Here's how the part is built. I have some questions about the finished solid (model axes, mm). A direction names the side the tool comes from. Give positions to 0.01 mm unless a question says otherwise; leave off trailing zeros. Write each loop counter-clockwise with the first axis right and the second up, starting at its lowest first coordinate (ties: lowest second). Pieces come first, ordered by that corner, then holes. Notation, with made-up numbers: (48.5, 70.25) - (53.5, 70.25) arc R24 ccw to (53.5, 105.25) - close; hole circle Ø9 at (-3, 46.25). An arc over 180 degrees is marked (long way). Use a Markdown table: item, result.
```python
from build123d import *

# Parameters (mm, degrees)
SKETCH1_W                  = 127.078191072
SKETCH1_H                  = 113.282646321
BOSS_EXTRUDE1_DEPTH        = 39.624
SHELL_1_T                  = -2.54
OFFICIAL_RIB_BLOCK20_REACH = 100.208


with BuildPart() as part:
    # Sketch1 → Boss-Extrude1 (new body)
    with BuildSketch(Plane(origin=(0, 0, 0), x_dir=(1, 0, 0), z_dir=(0, 1, 0))):
        with Locations((1.06119575, 7.295720781)):
            Rectangle(SKETCH1_W, SKETCH1_H)
    extrude(amount=BOSS_EXTRUDE1_DEPTH)

    # 抽壳1
    shell_1_openings = [part.faces().sort_by_distance(p)[0] for p in [
        (1.06119575, 39.624, -7.295720782),
    ]]
    offset(amount=SHELL_1_T, openings=shell_1_openings, kind=Kind.INTERSECTION)

    # 草图1 walls → official_rib_block20 (add, up to next)
    with BuildSketch(Plane(origin=(0.729572078, 0, -0.729572078), x_dir=(0.7071067811865477, 0, 0.7071067811865475), z_dir=(-0.7071067811865475, 0, 0.7071067811865477)), mode=Mode.PRIVATE) as official_rib_block20_sk1:
        Polygon((-181.514338156, -5.000960726), (-34.23, 35.134), (7.726, 25.357), (209.797270961, 53.134303954), (209.451367988, 55.650640802), (7.84521248, 27.93727297), (-34.278590113, 37.753375981), (-182.182137615, -2.550319201), align=None)
    official_rib_block20_tool1 = extrude(official_rib_block20_sk1.sketch, amount=-OFFICIAL_RIB_BLOCK20_REACH, mode=Mode.PRIVATE) - part.part
    add(official_rib_block20_tool1.solids().sort_by_distance((-8.641006986, 30.2455, -10.100151142))[0])


solid = part.part
```
Item 1: For faces 5 (the flat face through (64.6, 20, -7)), 6 (the flat face through (46.229, 28.993, 2.099)), 7 (the flat face through (-23.509, 32.392, -52.792)), which set-ups out of +Z, -Z, +X, -X, +Y, -Y let a thin tool reach every point of the face, with its end or its side?
Values:
| item | result |
|---|---|
| face 5 | +Z, -Z, +X, +Y, -Y |
| face 6 | none |
| face 7 | +Y |
Item 2: If we section it at D-D, the plane z = -17.5: Write out the boundary of the cut face in (x, y).
Values:
| item | result |
|---|---|
| outline | (-62.48, 0) - (64.6, 0) - (64.6, 39.62) - (62.06, 39.62) - (62.06, 31.19) - (28.59, 27.94) - (-16.04, 35.29) - (-16.04, 32.68) - (28.43, 25.36) - (62.06, 28.63) - (62.06, 2.54) - (-59.94, 2.54) - (-59.94, 39.62) - (-62.48, 39.62) - close |
Item 3: Will this pin go through, and if not, where does the flat tip stop? pin 1 Ø1 at (x, z) = (-26, -29) entering from +Y.
Values:
| item | result |
|---|---|
| pin 1 | stops at y = 36.63 |
Item 4: If we section it at A-A, the plane y = 7.5: Write out the boundary of the cut face in (x, z).
Values:
| item | result |
|---|---|
| outline | (-62.48, -63.94) - (64.6, -63.94) - (64.6, 49.35) - (-62.48, 49.35) - close; hole (-59.94, -61.4) - (62.06, -61.4) - (62.06, 46.81) - (-59.94, 46.81) - close |
Item 5: If we section it at B-B, the plane z = 9.5: Write out the boundary of the cut face in (x, y).
Values:
| item | result |
|---|---|
| outline | (-62.48, 0) - (64.6, 0) - (64.6, 39.62) - (62.06, 39.62) - (62.06, 33.81) - (10.96, 28.85) - (10.96, 26.28) - (62.06, 31.25) - (62.06, 2.54) - (-59.94, 2.54) - (-59.94, 39.62) - (-62.48, 39.62) - close |
Item 6: I need wall thicknesses on line 1 along X through (y, z) = (31, 42); line 2 along Z through (x, y) = (-19.5, 15.5); line 3 along Y through (x, z) = (5.5, 15). Which ranges of each line are inside material? Lowest first, please. Write a range as [from, to].
Values:
| item | result |
|---|---|
| line 1 | x = [-62.48, -59.94], [62.06, 64.6] |
| line 2 | z = [-63.94, -61.4], [46.81, 49.35] |
| line 3 | y = [0, 2.54] |
Item 7: If we section it at C-C, the plane x = 4: Write out the boundary of the cut face in (y, z).
Values:
| item | result |
|---|---|
| outline | (0, -63.94) - (39.62, -63.94) - (39.62, -61.4) - (36.03, -61.4) - (37.75, -52.48) - (28.69, 2.54) - (26.08, 2.54) - (35.13, -52.41) - (33.4, -61.4) - (2.54, -61.4) - (2.54, 46.81) - (39.62, 46.81) - (39.62, 49.35) - (0, 49.35) - close |
Item 8: Thinking about a two-plate mould opening in Z: for faces 1 (the flat face through (0, 2.54, -8)), 2 (the flat face through (-60.4, 39.624, -7.6)), 3 (the flat face through (0, 20, 49.346)), 4 (the flat face through (0, 20, -63.937)), which applies, +Z half, -Z half, draft (parallel to the pull), parting line (faces both ways), or undercut?
Values:
| item | result |
|---|---|
| face 1 | undercut |
| face 2 | draft |
| face 3 | +Z half |
| face 4 | -Z half |
